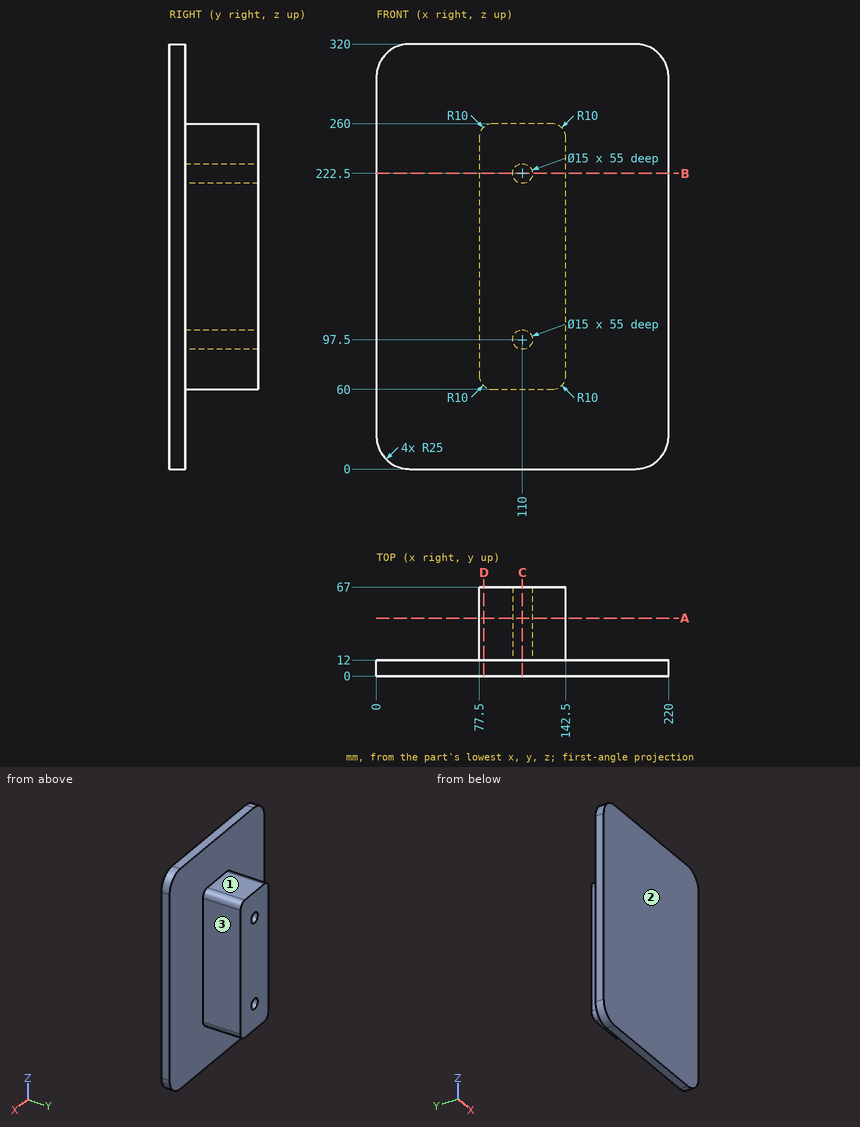
Geometry: see drawing. Coordinates: mm, zero at the bounding-box minimum. A direction names the side the tool comes from. Give positions to 0.01 mm unless a question says otherwise; leave off trailing zeros. Write each loop counter-clockwise with the first axis right and the second up, starting at its lowest first coordinate (ties: lowest second). Pieces come first, ordered by that corner, then holes. Notation, with made-up numbers: M 30,-27.5 L 60,-27.5 A24 cw 60,11.5 Z; hole C -36,22.25 d1. An arc over 180 degrees is marked long. Return JSON: item names as keys, results as strings. Group by question number.
1) Cut plane A-A, the plane y = 43.5. Output: boundary loops of the cut face in (x, z).
2) Cut plane B-B, the plane z = 222.5. Output: boundary loops of the cut face in (x, y).
3) Cut plane C-C, the plane x = 110. Output: boundary loops of the cut face in (y, z).
4) Ray query, L1, parallel to X at y = 48, z = 222.5; L2, parallel to X at y = 36.5, z = 96.5; L3, parallel to Y at x = 17, z = 159. Return the intervals inside material, ascending.
5) Cut plane D-D, the plane x = 81. Output: boundary loops of the cut face in (y, z), then the cut area to 3 significant figures.
6) Set-up query: the marked faces 1, 2 and 3. Return all of +Z, -Z, +X, -X, +Y, -Y with unobstructed straight access to the full face (end or side cutting, diameter ignored); none if empty.
7) First-contact query: pin 1 Ø4 at (x, z) = (38, 287.5) entering from +Y; pin 2 Ø7.5 at (x, z) = (106.5, 224.5) entering from +Y; pin 3 Ø8 at (x, y) = (149, 25.5) entering from +Z; pin 4 Ø6 at (y, z) = (50, 205.5) entering from +X. Flat tips, straight axial feed; report the tip coordinate or a pass-through.
Data:
{
 "1": {"outline": "M 77.5,70 A10 ccw 87.5,60 L 132.5,60 A10 ccw 142.5,70 L 142.5,250 A10 ccw 132.5,260 L 87.5,260 A10 ccw 77.5,250 Z; hole C 110,97.5 d15; hole C 110,222.5 d15"},
 "2": {"outline": "M 0,0 L 220,0 L 220,12 L 142.5,12 L 142.5,67 L 117.5,67 L 117.5,12 L 102.5,12 L 102.5,67 L 77.5,67 L 77.5,12 L 0,12 Z"},
 "3": {"outline": "M 0,0 L 12,0 L 12,60 L 67,60 L 67,90 L 12,90 L 12,105 L 67,105 L 67,215 L 12,215 L 12,230 L 67,230 L 67,260 L 12,260 L 12,320 L 0,320 Z"},
 "4": {"L1": "x = 77.5 to 102.5, 117.5 to 142.5", "L2": "x = 77.5 to 102.57, 117.43 to 142.5", "L3": "y = 0 to 12"},
 "5": {"outline": "M 0,0 L 12,0 L 12,62.4 L 67,62.4 L 67,257.6 L 12,257.6 L 12,320 L 0,320 Z", "area": "14,600 mm²"},
 "6": {"face 1": "+Z, +X, -X, +Y", "face 2": "+Z, -Z, +X, -X, -Y", "face 3": "+Z, -Z, +X, +Y"},
 "7": {"pin 1": "stops at y = 12", "pin 2": "stops at y = 67", "pin 3": "passes through", "pin 4": "stops at x = 142.5"}
}
